Here's how the part is built. I have some questions about the finished solid (model axes, mm). A direction names the side the tool comes from. Give positions to 0.01 mm unless a question says otherwise; leave off trailing zeros. Write each loop counter-clockwise with the first axis right and the second up, starting at its lowest first coordinate (ties: lowest second). Pieces come first, ordered by that corner, then holes. Notation, with made-up numbers: (-11.75, 37) -> (-0.75, 37) arc R10 ccw to (-0.75, 52) -> close; hole circle Ø3 at (1.25, -34.5). An arc over 180 degrees is marked (long way). Use one line per item in the form item = value.
```python
from build123d import *

# Parameters (mm, degrees)
SKETCH_1_R                  = 1.55
SKETCH_1_W                  = 8
SKETCH_1_H                  = 5
SKETCH_1_W_2                = 11
SKETCH_1_H_2                = 7.8
EXTRUDE_1_DEPTH             = 3
HOLE_WIZARD_M3_1_AT_2_COUNT = 2
HOLE_WIZARD_M3_1_AT_2_PITCH = 26
HOLE_WIZARD_M3_1_AT_3_COUNT = 2
HOLE_WIZARD_M3_1_AT_3_PITCH = 42.011903075
HOLE_WIZARD_M3_1_AT_4_COUNT = 2
HOLE_WIZARD_M3_1_AT_4_PITCH = 33
FILLET_1_R                  = 1


with BuildPart() as part:
    # 草图1 → 凸台-拉伸1 (new body)
    with BuildSketch(Plane(origin=(0, 0, 0), x_dir=(0, 0, -1), z_dir=(1, 0, 0))):
        Polygon((16.5, -18.9), (-16.5, -18.9), (-16.5, -18.7), (-31.5, -18.7), (-31.5, 6.3), (-16.5, 6.3), (-16.5, 18.9), (16.5, 18.9), (16.5, 6.3), (31.5, 6.3), (31.5, -18.7), (16.5, -18.7), align=None)
        with Locations((-13, 16.5)):
            Circle(SKETCH_1_R, mode=Mode.SUBTRACT)
        with Locations((-13, -16.5)):
            Circle(SKETCH_1_R, mode=Mode.SUBTRACT)
        with Locations(Location((13, -16.5, 0), (0, 0, 180))):
            Circle(SKETCH_1_R, mode=Mode.SUBTRACT)
        with Locations(Location((13, 16.5, 0), (0, 0, 180))):
            Circle(SKETCH_1_R, mode=Mode.SUBTRACT)
        with Locations((24.5, -10)):
            Rectangle(SKETCH_1_W, SKETCH_1_H, mode=Mode.SUBTRACT)
        with Locations((-24.5, -10)):
            Rectangle(SKETCH_1_W, SKETCH_1_H, mode=Mode.SUBTRACT)
        Polygon((-13.5, -11.378679656), (-2.121320344, 0), (-13.5, 11.378679656), align=None, mode=Mode.SUBTRACT)
        Polygon((-11.378679656, -13.5), (0, -2.121320344), (11.378679656, -13.5), align=None, mode=Mode.SUBTRACT)
        Polygon((-11.378679656, 13.5), (0, 2.121320344), (11.378679656, 13.5), align=None, mode=Mode.SUBTRACT)
        Polygon((13.5, 11.378679656), (13.5, -11.378679656), (2.121320344, 0), align=None, mode=Mode.SUBTRACT)
        with Locations((23, -0.6)):
            Rectangle(SKETCH_1_W_2, SKETCH_1_H_2, mode=Mode.SUBTRACT)
        with Locations((-23, -0.6)):
            Rectangle(SKETCH_1_W_2, SKETCH_1_H_2, mode=Mode.SUBTRACT)
    extrude(amount=EXTRUDE_1_DEPTH)

    # 草图2 → M3 锥坑高头螺钉的锥形沉头孔1 (revolve, cut)
    with BuildSketch(Plane(origin=(3, 16.5, 13), x_dir=(0, 0, -1), z_dir=(0, 1, 0))):
        Polygon((0, 0), (0, 3), (1.55, 3), (1.55, 1.6), (3.15, 0), align=None)
    hole_wizard_m3_1 = revolve(axis=Axis((9.35, 16.5, 13), (-1, 0, 0)), mode=Mode.SUBTRACT)

    # M3 锥坑高头螺钉的锥形沉头孔1 at 2: M3 锥坑高头螺钉的锥形沉头孔1 ×2
    with Locations(*[(0, 0, -i * HOLE_WIZARD_M3_1_AT_2_PITCH) for i in range(1, HOLE_WIZARD_M3_1_AT_2_COUNT)]):
        add(hole_wizard_m3_1, mode=Mode.SUBTRACT)

    # M3 锥坑高头螺钉的锥形沉头孔1 at 3: M3 锥坑高头螺钉的锥形沉头孔1 ×2
    with Locations(*[Vector(0, -0.7854916722275357, -0.6188722266035129) * (i * HOLE_WIZARD_M3_1_AT_3_PITCH) for i in range(1, HOLE_WIZARD_M3_1_AT_3_COUNT)]):
        add(hole_wizard_m3_1, mode=Mode.SUBTRACT)

    # M3 锥坑高头螺钉的锥形沉头孔1 at 4: M3 锥坑高头螺钉的锥形沉头孔1 ×2
    with Locations(*[(0, -i * HOLE_WIZARD_M3_1_AT_4_PITCH, 0) for i in range(1, HOLE_WIZARD_M3_1_AT_4_COUNT)]):
        add(hole_wizard_m3_1, mode=Mode.SUBTRACT)

    # 圆角1
    fillet_1_edges = [part.edges().sort_by_distance(p)[0] for p in [
        (1.5, 11.378679656, -13.5),
        (1.5, 0, -2.121320344),
        (1.5, -11.378679656, -13.5),
        (1.5, -12.5, 20.5),
        (1.5, -7.5, 20.5),
        (1.5, -7.5, 28.5),
        (1.5, -12.5, 28.5),
        (1.5, -12.5, -28.5),
        (1.5, -7.5, -28.5),
        (1.5, -7.5, -20.5),
        (1.5, -12.5, -20.5),
        (1.5, 11.378679656, 13.5),
        (1.5, -11.378679656, 13.5),
        (1.5, 0, 2.121320344),
        (1.5, 2.121320344, 0),
        (1.5, 13.5, -11.378679656),
        (1.5, 13.5, 11.378679656),
        (1.5, -13.5, 11.378679656),
        (1.5, -13.5, -11.378679656),
        (1.5, -2.121320344, 0),
    ]]
    fillet(fillet_1_edges, radius=FILLET_1_R)


solid = part.part
```
Q1. If we mould it in two halves opening along Z, with no side actions, what happens to faces 1 (the face through (1, -1, -17.5)), 2 (the face through (1, 6.3, 24))? For each: +Z half, -Z half, draft (parallel to the pull), parting line (faces both ways), or undercut.
Result set:
face_1 = undercut
face_2 = draft
Q2. Will these pins go through, and if not, where does the flat tip stop? pin 1 Ø1.5 at (x, z) = (2, 25) entering from -Y; pin 2 Ø1.9 at (y, z) = (-16.5, -13) entering from -X; pin 3 Ø1.5 at (x, y) = (1, 11) entering from +Z.
Result set:
pin_1 = -18.7
pin_2 = through
pin_3 = 16.5
Q3. I want a section at C-C, the plane z = -1.5. Write out the boundary of the cut face in (x, y), and give its area (3 significant figures).
Result set:
outline = (0, -18.9) -> (3, -18.9) -> (3, -13.5) -> (0, -13.5) -> close; (0, -3.62) -> (3, -3.62) -> (3, 3.62) -> (0, 3.62) -> close; (0, 13.5) -> (3, 13.5) -> (3, 18.9) -> (0, 18.9) -> close
area = 54.1 mm2
Q4. I want a section at A-A, the plane y = -16.5. Write out the boundary of the cut face in (x, z).
Result set:
outline = (0, -31.5) -> (3, -31.5) -> (3, -16.15) -> (1.4, -14.55) -> (0, -14.55) -> close; (0, -11.45) -> (1.4, -11.45) -> (3, -9.85) -> (3, 9.85) -> (1.4, 11.45) -> (0, 11.45) -> close; (0, 14.55) -> (1.4, 14.55) -> (3, 16.15) -> (3, 31.5) -> (0, 31.5) -> close
Q5. I want a section at B-B, the plane y = 4. Write out the boundary of the cut face in (x, z), and give its area (3 significant figures).
Result set:
outline = (0, -31.5) -> (3, -31.5) -> (3, -13.5) -> (0, -13.5) -> close; (0, -6.12) -> (3, -6.12) -> (3, -1.88) -> (0, -1.88) -> close; (0, 1.88) -> (3, 1.88) -> (3, 6.12) -> (0, 6.12) -> close; (0, 13.5) -> (3, 13.5) -> (3, 31.5) -> (0, 31.5) -> close
area = 133 mm2
Q6. I want a section at D-D, the plane y = 16.5. Write out the boundary of the cut face in (x, z).
Result set:
outline = (0, -16.5) -> (3, -16.5) -> (3, -16.15) -> (1.4, -14.55) -> (0, -14.55) -> close; (0, -11.45) -> (1.4, -11.45) -> (3, -9.85) -> (3, 9.85) -> (1.4, 11.45) -> (0, 11.45) -> close; (0, 14.55) -> (1.4, 14.55) -> (3, 16.15) -> (3, 16.5) -> (0, 16.5) -> close
Q7. Which directions (+Z, -Z, +X, -X, +Y, -Y) give clear straight access to the entire face, cutting with the end or side of a thin tool? Please do faces 3 (the face through (1.52, 9.88, -12.9)), 4 (the face through (1.678, -14.716, 13.396)).
Result set:
face_3 = +X, -X
face_4 = +X
Q8. If I drill on line 1 along Z through (x, y) = (0.9, 16.5); line 2 along Y through (x, z) = (2.5, 25.5); line 3 along Z through (x, y) = (0.85, -16.5), over which ranges is the centre line in solid material (lowest first)? Write a range as from..to.
Result set:
line_1 = -16.5..-14.55, -11.45..11.45, 14.55..16.5
line_2 = -18.7..-12.5, -7.5..-4.5, 3.3..6.3
line_3 = -31.5..-14.55, -11.45..11.45, 14.55..31.5
